For this review, take the finished solid that the model builds, in its own axes (mm). A direction names the side the tool comes from. Coordinates: 2 decimals unless noted, no trailing zeros. Write each loop counter-clockwise with the first axis right and the second up, starting at its lowest first coordinate (ties: lowest second). Pieces come first, ordered by that corner, then holes. Notation, with made-up numbers: M 55.25,18 L 104.25,18 A17 ccw 104.25,36 Z; hole C 35.25,-13.75 d10. An arc over 180 degrees is marked long. Return JSON: item names as keys, results as strings.
```python
from build123d import *

# Parameters (mm, degrees)
SKETCH1_W                = 30
SKETCH1_H                = 30
BOSS_EXTRUDE1_DEPTH      = 3.82
CUT_EXTRUDE2_DEPTH       = 43.598032818
CUT_EXTRUDE5_DEPTH       = 45
BOSS_EXTRUDE2_DEPTH      = 10
BOSS_EXTRUDE2_DEPTH_BACK = 5
SKETCH4_R                = 0.875
BOSS_EXTRUDE3_DEPTH      = 10
BOSS_EXTRUDE3_DEPTH_BACK = 5
SKETCH5_R                = 0.875


with BuildPart() as part:
    # Sketch1 → Boss-Extrude1 (new body)
    with BuildSketch(Plane(origin=(0, 0, 0), x_dir=(1, 0, 0), z_dir=(0, 1, 0))):
        with Locations((15, 15)):
            Rectangle(SKETCH1_W, SKETCH1_H)
    extrude(amount=BOSS_EXTRUDE1_DEPTH)

    # Sketch2 → Cut-Extrude2 (cut, through all)
    with BuildSketch(Plane.XY):
        Polygon((-3, 1.91), (0, 1.91), (0, 3.82), align=None)
        with BuildLine():
            ThreePointArc((0, 3.82), (0.556416736, 1.91), (0, 0))
            Line((0, 0), (0, 3.82))
        make_face()
        Polygon((0, 0), (0, 1.91), (-3, 1.91), align=None)
        Polygon((30, 3.82), (30, 1.91), (43, 1.91), align=None)
        Polygon((43, 1.91), (30, 1.91), (30, 0), align=None)
        with BuildLine():
            ThreePointArc((30, 3.82), (29.860437602, 1.91), (30, 0))
            Line((30, 0), (30, 3.82))
        make_face()
    extrude(amount=-CUT_EXTRUDE2_DEPTH, mode=Mode.SUBTRACT)

    # Sketch3 → Cut-Extrude5 (cut)
    with BuildSketch(Plane(origin=(0, 0, 0), x_dir=(0, 0, -1), z_dir=(1, 0, 0))):
        with BuildLine():
            Line((30, 3.82), (43, 1.91))
            Line((43, 1.91), (30, 0))
            ThreePointArc((30, 0), (29.860437602, 1.91), (30, 3.82))
        make_face()
        with BuildLine():
            Line((0, 3.82), (-13, 1.91))
            Line((-13, 1.91), (0, 0))
            ThreePointArc((0, 0), (0.139562398, 1.91), (0, 3.82))
        make_face()
    extrude(amount=CUT_EXTRUDE5_DEPTH, mode=Mode.SUBTRACT)

    # Sketch4 → Boss-Extrude2 (add, two sides: drawn at the far end of the back side and taken through both)
    with BuildSketch(Plane.XY.offset(-BOSS_EXTRUDE2_DEPTH_BACK)):
        with Locations((2.5, 1.91)):
            Circle(SKETCH4_R)
    extrude(amount=BOSS_EXTRUDE2_DEPTH + BOSS_EXTRUDE2_DEPTH_BACK)

    # Sketch5 → Boss-Extrude3 (add, two sides: drawn at the far end of the back side and taken through both)
    with BuildSketch(Plane.XY.offset(-BOSS_EXTRUDE3_DEPTH_BACK)):
        with Locations((27.410666516, 1.91)):
            Circle(SKETCH5_R)
    extrude(amount=BOSS_EXTRUDE3_DEPTH + BOSS_EXTRUDE3_DEPTH_BACK)


solid = part.part
```
1. Draft analysis for pull direction Y (two halves, no side actions). For faces 1 (the face through (27, 2, 10)), 2 (the face through (15, 0, -15)), 3 (the face through (0.556, 1.938, -14.79)), state which applies: +Y half, -Y half, draft (parallel to the pull), parting line (faces both ways), or undercut.
Checks:
{"face 1": "draft", "face 2": "-Y half", "face 3": "undercut"}
2. For faces 4 (the face through (15, 3.82, -15)), 5 (the face through (28.219, 1.575, 4.859)), list the 3-axis set-ups (+Z, -Z, +X, -X, +Y, -Y) from which the entire face can be reached by the end or side of a thin tool; tool diameter is ignored.
Checks:
{"face 4": "+Z, -Z, +X, -X, +Y", "face 5": "+Z"}
3. We need section A-A (y = 1.91). State the section outline as (x, z) points (3 decimals).
Checks:
{"outline": "M 0.556,-29.86 L 29.86,-29.86 L 29.86,-0.14 L 28.286,-0.14 L 28.286,10 L 26.536,10 L 26.536,-0.14 L 3.375,-0.14 L 3.375,10 L 1.625,10 L 1.625,-0.14 L 0.556,-0.14 Z"}
4. Wall thickness on L1, parallel to X at y = 2.15, z = -5; L2, parallel to Z at x = 28, y = 2.3; L3, parallel to Z at x = 17, y = 2.1: over which ranges is each line inside the solid? List them lowest first. Write a range as from..to.
Checks:
{"L1": "0.55..29.86", "L2": "-29.87..10", "L3": "-29.86..-0.14"}
5. We need section B-B (z = 7.5). State the section outline as (x, y) points (3 decimals).
Checks:
{"outline": "C 2.5,1.91 d1.75; C 27.411,1.91 d1.75"}
6. Clearance check with a flat-ended pin moving along its axis: pin 1 Ø1 at (x, y) = (3, 2) entering from -Z. State where the tip first meets the part, or that it passes through.
Checks:
{"pin 1": "z = -29.87"}
7. We need section D-D (z = -10). State the section outline as (x, y) points, plus the area to 3 significant figures.
Checks:
{"outline": "M 0,0 L 30,0 A13.14 cw 30,3.82 L 0,3.82 A3.56 cw Z", "area": "113 mm2"}
8. We need section C-C (x = 2.5). State the section outline as (y, z) points (3 decimals).
Checks:
{"outline": "M 0,-30 A13.14 cw 3.82,-30 L 3.82,0 A13.14 cw 2.785,-0.11 L 2.785,10 L 1.035,10 L 1.035,-0.11 A13.14 cw 0,0 Z"}
